```python
from build123d import *

# Parameters (mm, degrees)
F0_W     = 85
F0_H     = 19.05
F1_DEPTH = 3.175
F3_R     = 4.75
F3_R_2   = 1.5
F4_DEPTH = 21.8
F2_R     = 1.5
F5_DEPTH = 15


with BuildPart() as f1:
    # F0 (on Front) → F1 (new body, symmetric)
    with BuildSketch(Plane.XZ):
        Rectangle(F0_W, F0_H)
    extrude(amount=F1_DEPTH, both=True)

    # F3 (on Front) → F4 (cut)
    with BuildSketch(Plane.XZ):
        with Locations((32.5, 0)):
            Circle(F3_R)
        with Locations((-19.5, 0)):
            Circle(F3_R_2)
    extrude(amount=F4_DEPTH, mode=Mode.SUBTRACT)

    # F2 (on Top) → F5 (cut)
    with BuildSketch(Plane.XY):
        with Locations((-25.5, 0)):
            Circle(F2_R)
        with Locations((25.5, 0)):
            Circle(F2_R)
    extrude(amount=-F5_DEPTH, mode=Mode.SUBTRACT)


solid = f1.part
```
Check sheet for the modelled part. Datum: model origin and axes. Units: mm. A direction names the side the tool comes from. Coordinates: 2 decimals unless noted, no trailing zeros. Loops run counter-clockwise (first coordinate to the right, second up) from the corner with the lowest first, then second, coordinate; pieces in that order, holes last.
1) Sectioned sample at D-D (z = -3.25). Record the boundary of the cut face in (x, y) (3 decimals), and give its area (3 significant figures).
2) Sectioned sample at C-C (x = -25.5). Record the boundary of the cut face in (y, z) (3 decimals).
3) Access from +Z, -Z, +X, -X, +Y, -Y to the whole of each face (thin tool, end or side, straight path). Record for faces 4 (the face through (-1, 3.175, 0)), 5 (the face through (25, 0, 0)), 6 (the face through (-20, 0, 0)).
4) Sectioned sample at B-B (x = 32.5). Record the boundary of the cut face in (y, z) (3 decimals), and give its area (3 significant figures).
5) Release check for a two-part mould opening along X. For faces 1 (the face through (42.5, 0, 0)), 2 (the face through (24, 0, -5)), 3 (the face through (-1, 0, 9.525)) record: released by +X, released by -X, zero draft, split by the parting line, or undercut.
6) Material ranges on probe 1 along X at (y, z) = (-2.2, 0); probe 2 along Z at (x, y) = (32.5, -1.55) (3 decimals); probe 3 along Y at (x, z) = (25.5, -2) (3 decimals), recorded low to high.
7) Gauge pin test, flat ends, axial feed: pin 1 (2.5 mm diameter, centred on x = -19.5, z = 0, fed in from -Y); pin 2 (1.5 mm diameter, centred on x = -26, y = -0.5, fed in from -Z); pin 3 (3.5 mm diameter, centred on x = -19, z = 0, fed in from -Y) (3 decimals). Record the tip position at first contact, or that the pin passes through.
8) Sectioned sample at A-A (z = -7). Record the boundary of the cut face in (x, y) (3 decimals).
Check sheet entries:
1. outline: (-42.5, -3.175) - (29.036, -3.175) - (29.036, 0) - (35.964, 0) - (35.964, -3.175) - (42.5, -3.175) - (42.5, 3.175) - (-42.5, 3.175) - close; hole circle Ø3 at (-25.5, 0); hole circle Ø3 at (25.5, 0)
1. area: 504 mm2
2. outline: (-3.175, -9.525) - (-1.5, -9.525) - (-1.5, 0) - (1.5, 0) - (1.5, -9.525) - (3.175, -9.525) - (3.175, 9.525) - (-3.175, 9.525) - close
3. face 4: +Z, -Z, +X, -X, +Y
3. face 5: -Z
3. face 6: -Y
4. outline: (-3.175, -9.525) - (3.175, -9.525) - (3.175, 9.525) - (-3.175, 9.525) - (-3.175, 4.75) - (0, 4.75) - (0, -4.75) - (-3.175, -4.75) - close
4. area: 90.8 mm2
5. face 1: released by +X
5. face 2: undercut
5. face 3: zero draft
6. probe 1: x = -42.5 to -21, -18 to 27.75, 37.25 to 42.5
6. probe 2: z = -9.525 to -4.75, 4.75 to 9.525
6. probe 3: y = -3.175 to -1.5, 1.5 to 3.175
7. pin 1: stops at y = 0
7. pin 2: stops at z = 0
7. pin 3: stops at y = -3.175
8. outline: (-42.5, -3.175) - (42.5, -3.175) - (42.5, 3.175) - (-42.5, 3.175) - close; hole circle Ø3 at (-25.5, 0); hole circle Ø3 at (25.5, 0)
